```python
from build123d import *

# Parameters (mm, degrees)
SALIENTE_EXTRUIR1_DEPTH      = 3.75
S_LIDO_MOVER_COPIAR2_ANGLE   = 180
S_LIDO_MOVER_COPIAR4_START   = -243.75
S_LIDO_MOVER_COPIAR4_DEPTH   = 7.5
S_LIDO_MOVER_COPIAR4_START_2 = -203.75
S_LIDO_MOVER_COPIAR4_2_DEPTH = 7.5
S_LIDO_MOVER_COPIAR4_START_3 = -123.75
S_LIDO_MOVER_COPIAR4_3_DEPTH = 7.5
S_LIDO_MOVER_COPIAR4_START_4 = -83.75
S_LIDO_MOVER_COPIAR4_4_DEPTH = 7.5
S_LIDO_MOVER_COPIAR5_ANGLE   = 124
S_LIDO_MOVER_COPIAR6_ANGLE   = 120
CROQUIS5_R                   = 6
SALIENTE_EXTRUIR4_DEPTH      = 275
SALIENTE_EXTRUIR5_START      = 86
CROQUIS6_R                   = 6
SALIENTE_EXTRUIR5_DEPTH      = 86
CROQUIS7_R                   = 6
SALIENTE_EXTRUIR6_DEPTH      = 26.25


# Read off the part's stored shape, not the designer's step: Sólido-Mover/Copiar4
with BuildPart() as part:
    # Croquis1 → Saliente-Extruir1 (new, symmetric)
    with BuildSketch(Plane.XY):
        with BuildLine():
            Line((-5.555796523, 15.775), (-10.936607328, 6.053149606))
            ThreePointArc((-10.936607328, 6.053149606), (0, -12.5), (10.936607328, 6.053149606))
            Line((10.936607328, 6.053149606), (5.555796523, 15.775))
            ThreePointArc((5.555796523, 15.775), (0, 19.05), (-5.555796523, 15.775))
        make_face()
    extrude(amount=SALIENTE_EXTRUIR1_DEPTH, both=True)


with BuildPart() as body_2:
    # Sólido-Mover/Copiar1: copy of part
    add(part.part.moved(Location((0, 0, 40))))


with BuildPart() as body_2_1:
    # Sólido-Mover/Copiar2: moved
    add(body_2.part.rotate(Axis((0, 0, 0), (0, 0, 1)), S_LIDO_MOVER_COPIAR2_ANGLE))


with BuildPart() as body_3:
    # Sólido-Mover/Copiar4 outline → Sólido-Mover/Copiar4 (new body)
    with BuildSketch(Plane.XY.offset(S_LIDO_MOVER_COPIAR4_START)):
        with BuildLine():
            ThreePointArc((5.555796523, 15.775), (0, 19.05), (-5.555796523, 15.775))
            Line((-5.555796523, 15.775), (-10.936607328, 6.053149606))
            ThreePointArc((-10.936607328, 6.053149606), (-12.5, 0), (-10.936607328, -6.053149606))
            ThreePointArc((-10.936607328, -6.053149606), (0, -12.5), (10.936607328, -6.053149606))
            ThreePointArc((10.936607328, -6.053149606), (12.5, 0), (10.936607328, 6.053149606))
            Line((10.936607328, 6.053149606), (5.555796523, 15.775))
        make_face()
    extrude(amount=S_LIDO_MOVER_COPIAR4_DEPTH)


with BuildPart() as body_4:
    # S_lido-Mover_Copiar4 2 outline → S_lido-Mover_Copiar4 2 (new body)
    with BuildSketch(Plane.XY.offset(S_LIDO_MOVER_COPIAR4_START_2)):
        with BuildLine():
            Line((-10.936607328, -6.053149606), (-5.555796523, -15.775))
            ThreePointArc((-5.555796523, -15.775), (0, -19.05), (5.555796523, -15.775))
            Line((5.555796523, -15.775), (10.936607328, -6.053149606))
            ThreePointArc((10.936607328, -6.053149606), (0, 12.5), (-10.936607328, -6.053149606))
        make_face()
    extrude(amount=S_LIDO_MOVER_COPIAR4_2_DEPTH)


with BuildPart() as body_5:
    # S_lido-Mover_Copiar4 3 outline → S_lido-Mover_Copiar4 3 (new body)
    with BuildSketch(Plane.XY.offset(S_LIDO_MOVER_COPIAR4_START_3)):
        with BuildLine():
            ThreePointArc((5.555796523, 15.775), (0, 19.05), (-5.555796523, 15.775))
            Line((-5.555796523, 15.775), (-10.936607328, 6.053149606))
            ThreePointArc((-10.936607328, 6.053149606), (-12.5, 0), (-10.936607328, -6.053149606))
            ThreePointArc((-10.936607328, -6.053149606), (0, -12.5), (10.936607328, -6.053149606))
            ThreePointArc((10.936607328, -6.053149606), (12.5, 0), (10.936607328, 6.053149606))
            Line((10.936607328, 6.053149606), (5.555796523, 15.775))
        make_face()
    extrude(amount=S_LIDO_MOVER_COPIAR4_3_DEPTH)


with BuildPart() as body_6:
    # S_lido-Mover_Copiar4 4 outline → S_lido-Mover_Copiar4 4 (new body)
    with BuildSketch(Plane.XY.offset(S_LIDO_MOVER_COPIAR4_START_4)):
        with BuildLine():
            Line((-10.936607328, -6.053149606), (-5.555796523, -15.775))
            ThreePointArc((-5.555796523, -15.775), (0, -19.05), (5.555796523, -15.775))
            Line((5.555796523, -15.775), (10.936607328, -6.053149606))
            ThreePointArc((10.936607328, -6.053149606), (0, 12.5), (-10.936607328, -6.053149606))
        make_face()
    extrude(amount=S_LIDO_MOVER_COPIAR4_4_DEPTH)


with BuildPart() as body_6_1:
    # Sólido-Mover/Copiar5: moved
    add(body_6.part.rotate(Axis((0, 0, 0), (0, 0, 1)), S_LIDO_MOVER_COPIAR5_ANGLE))


with BuildPart() as body_5_1:
    # Sólido-Mover/Copiar5: moved
    add(body_5.part.rotate(Axis((0, 0, 0), (0, 0, 1)), S_LIDO_MOVER_COPIAR5_ANGLE))


with BuildPart() as body_3_1:
    # Sólido-Mover/Copiar6: moved
    add(body_3.part.rotate(Axis((0, 0, 0), (0, 0, -1)), S_LIDO_MOVER_COPIAR6_ANGLE))


with BuildPart() as body_4_1:
    # Sólido-Mover/Copiar6: moved
    add(body_4.part.rotate(Axis((0, 0, 0), (0, 0, -1)), S_LIDO_MOVER_COPIAR6_ANGLE))


with BuildPart() as part_1:
    add(part.part)

    add(body_2_1.part)  # Saliente-Extruir4 merges body 2

    add(body_3_1.part)  # Saliente-Extruir4 merges body 3

    add(body_4_1.part)  # Saliente-Extruir4 merges body 4

    add(body_5_1.part)  # Saliente-Extruir4 merges body 5

    add(body_6_1.part)  # Saliente-Extruir4 merges body 6
    # Croquis5 → Saliente-Extruir4 (add)
    with BuildSketch(Plane.XY.offset(-236.25)):
        Circle(CROQUIS5_R)
    extrude(amount=SALIENTE_EXTRUIR4_DEPTH)

    # Croquis6 → Saliente-Extruir5 (add)
    with BuildSketch(Plane(origin=(0, 0, -243.75), x_dir=(-1, 0, 0), z_dir=(0, 0, -1)).offset(SALIENTE_EXTRUIR5_START)):
        with Locations(Location((0, 0, 0), (0, 0, 180))):
            Circle(CROQUIS6_R)
    extrude(amount=-SALIENTE_EXTRUIR5_DEPTH)

    # Croquis7 → Saliente-Extruir6 (add)
    with BuildSketch(Plane.XY.offset(43.75)):
        Circle(CROQUIS7_R)
    extrude(amount=SALIENTE_EXTRUIR6_DEPTH)


solid = part_1.part
```
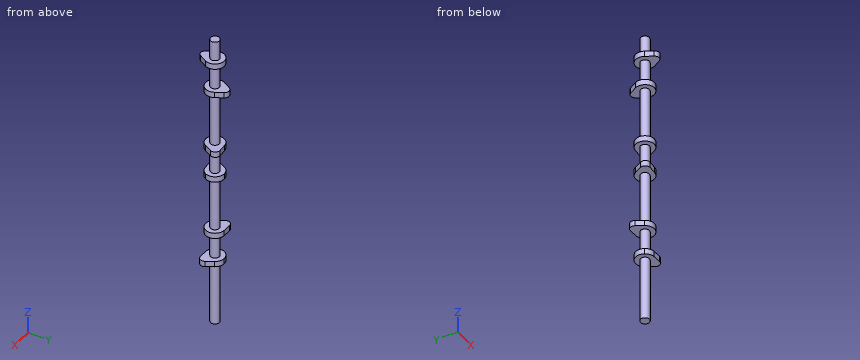
Geometry check sheet. Reference: the model listing, model coordinates, mm. Give positions to 0.01 mm unless a question says otherwise; leave off trailing zeros. Write each loop counter-clockwise with the first axis right and the second up, starting at its lowest first coordinate (ties: lowest second). Pieces come first, ordered by that corner, then holes. Notation, with made-up numbers: (36, 4) -> (55, 4) arc R14 cw to (55, 10) -> close; hole circle Ø4 at (30.5, 61.5). An arc over 180 degrees is marked (long way). One line per question, with ' | ' between items.
Item 1: Depth check by flat-ended pin: pin 1 (2 mm diameter, centred on x = 3.5, z = -140, fed in from +Y); pin 2 (6 mm diameter, centred on x = 2, z = -8, fed in from -Y); pin 3 (6 mm diameter, centred on x = -1, z = -234, fed in from +Y). Enter the tip coordinate at first touch or a pass-through.
Determined:
pin 1: y = 5.45 | pin 2: y = -6 | pin 3: y = 12.5
Item 2: Sectioned sample at A-A, the plane z = -227. Record the boundary of the cut face in (x, y).
Determined:
outline: circle Ø12 at (0, 0)
Item 3: Scan lines: line 1 along Z through (x, y) = (-1, -10); line 2 along X through (y, z) = (0, -153); line 3 along Z through (x, y) = (-13.5, 11). Record each from-to range of solid material in increasing order.
Determined:
line 1: -243.75 to -236.25, -203.75 to -196.25, -123.75 to -116.25, -83.75 to -76.25, -3.75 to 3.75, 36.25 to 43.75 | line 2: -6 to 6 | line 3: -203.75 to -196.25
